Autodesk Inventor part; units mm, degrees
ref_plane "Work Plane1" through (-9, 0, 0) normal (1, 0, 0) x (0, 0, -1)
ref_plane "Work Plane2" through (-3.5, 4, 0) normal (0, 1, 0) x (1, 0, 0)
ref_plane "YZ Plane" through (0, 0, 0) normal (1, 0, 0) x (0, 1, 0)
sketch "Sketch1" plane through (0, 0, 0) normal (0, 1, 0) x (-1, 0, 0)
  line L0 (0, 0) -> (18, 0)
  line L1 (18, 0) -> (18, -4)
  line L2 (18, -4) -> (0, -4)
  line L3 (0, -4) -> (0, 0)
  line L4 (18, -2) -> (16, -2)
  line L5 (9, -4) -> (9, -3)
  circle A0 centre (16, -2) radius 1.1
  circle A1 centre (2, -2) radius 1.1
  dimension "d0" = 18
  dimension "d1" = 4
  dimension "d2" = 2
  dimension "d3" = 2.2
extrude "Extrusion1" add sketch "Sketch1" along normal blind 8 contours A0 | L0 L1 L2 L3 | A1
sketch "Sketch2" plane through (0, 0, -4) normal (0, 0, -1) x (-1, 0, 0)
  line L0 (18, 0) -> (18, 8)
  line L1 (18, 8) -> (18, 6.1)
  line L2 (18, 0) -> (0, 0)
  line L3 (18, 0) -> (18, 1.9)
  line L4 (18, 6.1) -> (14.5, 6.1)
  line L5 (14.5, 6.1) -> (14.5, 1.9)
  line L6 (14.5, 1.9) -> (18, 1.9)
  line L7 (18, 1.9) -> (18, 6.1)
  dimension "d6" = 1.9
  dimension "d7" = 1.9
  dimension "d8" = 3.5
extrude "Extrusion2" cut sketch "Sketch2" against normal blind 8
ref_plane "Work Plane1" through (-9, 0, 0) normal (1, 0, 0) x (0, 0, -1)
mirror "Mirror1" about plane through (-9, 0, 0) normal (1, 0, 0) of "Extrusion2"
extrude "Extrusion3" cut sketch "Sketch1" along normal blind 8 contours A0 | A1
sketch "Sketch4" plane through (0, 8, 0) normal (0, 1, 0) x (1, 0, 0)
  line L0 (-18, 0) -> (0, 0)
  line L1 (0, 0) -> (-4, 0)
  line L2 (-4, 0) -> (-4, 4)
  line L3 (-4, 4) -> (0, 4)
  line L4 (0, 4) -> (0, 0)
  circle A0 centre (-2, 2) radius 1.1
  circle A1 centre (-2, 2) radius 1.1
  dimension "d14" = 4
  dimension "d15" = 4
  dimension "d16" = 2.2
extrude "Extrusion4" add sketch "Sketch4" along normal blind 3.25
ref_plane "Work Plane2" through (-3.5, 4, 0) normal (0, 1, 0) x (1, 0, 0)
mirror "Mirror2" about plane through (-3.5, 4, 0) normal (0, 1, 0) of "Extrusion4"
fillet "Fillet2" radius 2 8 edges at (0, 8.675, -4) (0, -0.675, -4) (0, -0.675, 0) (0, 8.675, 0) (-18, 7.05, -4) (-18, 0.95, -4) (-18, 7.05, 0) (-18, 0.95, 0)
chamfer "Chamfer1" distance 3.25 angle 45 2 edges at (-4, 8, -2) (-4, 0, -2)
sketch "Sketch5" plane through (-14.5, 1.9, 0) normal (0, 0, 1) x (1, 0, 0)
  line L0 (0, 0) -> (-1.5, 0)
  line L1 (0, 0) -> (-4.1729, 0)
  line L2 (-4.1729, 0) -> (-4.1729, 7.3414)
  line L3 (-4.1729, 7.3414) -> (0, 7.3414)
  line L4 (0, 7.3414) -> (0, 0)
  line L5 (0, 0) -> (-4.2733, 0)
  line L6 (-4.2733, 0) -> (-4.2733, -4.4882)
  line L7 (-4.2733, -4.4882) -> (0, -4.4882)
  line L8 (0, -4.4882) -> (0, 0)
  point P0 (14.5, -1.9)
extrude "Extrusion5" cut sketch "Sketch5" against normal blind 10
sketch "Sketch6" plane through (0, 0, 0) normal (0, -1, 0) x (1, 0, 0)
  line L0 (-14.5, 0) -> (-14.5, -4)
  line L1 (-14.5, -2) -> (-16, -2)
  line L2 (-14.5, 0) -> (-7.25, 0)
  line L3 (-7.25, -4) -> (-14.5, -4)
  line L4 (-14.5, 0) -> (-12.5, 0)
  line L5 (-12.5, 0) -> (-12.5, -4)
  line L6 (-12.5, -4) -> (-14.5, -4)
  line L7 (-14.5, -4) -> (-14.5, 0)
  point P0 (0, 0)
  dimension "d25" = 1.5
  dimension "d26" = 2
extrude "Extrusion6" cut sketch "Sketch6" against normal blind 10
sketch "Sketch7" plane through (0, 0, 0) normal (0, -1, 0) x (1, 0, 0)
  line L0 (-12.5, 0) -> (-12.5, -4)
  line L1 (-12.5, -2) -> (-16, -2)
  line L2 (-12.5, 0) -> (-7.25, 0)
  line L3 (-16, -2) -> (-12.5, 0)
  line L4 (-7.25, -4) -> (-12.5, -4)
  line L5 (-12.5, 0) -> (-12.5, -4)
  line L6 (-12.5, -4) -> (-16, -2)
  point P0 (0, 0)
  dimension "d29" = 3.5
extrude "Extrusion7" add sketch "Sketch7" against normal blind 8
properties part number "short_link_v3"
Work out the finished part from the listing and answer in its coordinate system (mm). A direction names the side the tool comes from. Give positions to 0.01 mm unless a question says otherwise; leave off trailing zeros. Loops run counter-clockwise (first coordinate to the right, second up) from the corner with the lowest first, then second, coordinate; pieces in that order, holes last. Notation, with made-up numbers: (83.25, -35) - (94.25, -35) arc R22 ccw to (94.25, -13) - close; hole circle Ø7 at (49.25, 29). An arc over 180 degrees is marked (long way). Answer in a Markdown table with one row per item. Add a question column.
Q1. The part is cut by section C-C (x = -7.5). Determine the outline of the cut face in (y, z), and give its area (3 significant figures).
Q2. Each of these flat-tipped pins is pushed along its axis until it touches: P1, Ø2, axis at x = -11.5, z = -2, coming from the -Y side; P2, Ø1.5, axis at x = -7.5, y = 8.5, coming from the +Z side; P3, Ø1.8, axis at x = -2, z = -2, coming from the -Y side; P4, Ø1.5, axis at y = 5.5, z = -0.5, coming from the +X side. Where does it stop, or does it pass through?
Q3. The part is cut by section D-D (x = -13). Determine the outline of the cut face in (y, z), and give its area (3 significant figures).
Q4. A tool of negligible diameter and unlimited length cuts with its end or side. For faces 1 (the flat face through (-11, 8, -2)), 2 (the flat face through (-11, 0, -2)), 3 (the flat face through (-3, 11.25, -1)), 4 (the flat face through (-3.5, 4, -2)), 5 (the flat face through (-14.27, 3.94, -1.01)), from which of +Z, -Z, +X, -X, +Y, -Y can it reach the whole face along a straight path? Write none if from no direction.
Q5. Consider line 1 along Z through (x, y) = (-2, 0.75); line 2 along Y through (x, z) = (-9.75, -1); line 3 along X through (y, z) = (10.4, -2). Determine where each line is inside the solid, lowest interval first.
Q6. Determine the mould class of faces 6 (the cylindrical face through (-0.6, 8.71, -0.57)), 7 (the flat face through (-5.65, 9.6, -2.03)), 8 (the flat face through (-1, 6.1, -3)), 9 (the flat face through (-1, 1.9, -3)) for opening direction Y: released by +Y, released by -Y, zero draft, split by the parting line, or undercut.
Q7. The part is cut by section A-A (z = -2.5). State how many separate pieces and enclosed holes the cut face has, and give its area (3 significant figures).
Q8. The part is cut by section B-B (y = 3). Determine the outline of the cut face in (x, z).
Solution:
| question | item | result |
|---|---|---|
| 1 | outline | (0, -4) - (8, -4) - (8, 0) - (0, 0) - close |
| 1 | area | 32.0 mm² |
| 2 | P1 | stops at y = 0 |
| 2 | P2 | stops at z = 0 |
| 2 | P3 | passes through |
| 2 | P4 | stops at x = -0.3 |
| 3 | outline | (0, -3.71) - (8, -3.71) - (8, -0.29) - (0, -0.29) - close |
| 3 | area | 27.4 mm² |
| 4 | face 1 | +Z, -Z, -X, +Y |
| 4 | face 2 | +Z, -Z, -X, -Y |
| 4 | face 3 | +Z, -Z, +X, -X, +Y |
| 4 | face 4 | +Z, -Z, +X |
| 4 | face 5 | +Z, -X, +Y, -Y |
| 5 | line 1 | z = -4 to -3.1, -0.9 to 0 |
| 5 | line 2 | y = 0 to 8 |
| 5 | line 3 | x = -4.85 to -3.1, -0.9 to 0 |
| 6 | face 6 | zero draft |
| 6 | face 7 | released by +Y |
| 6 | face 8 | undercut |
| 6 | face 9 | undercut |
| 7 | separate pieces | 3 |
| 7 | enclosed holes | 0 |
| 7 | area | 122 mm² |
| 8 | outline | (-16, -2) - (-12.5, -4) - (-3.5, -4) - (-3.5, 0) - (-12.5, 0) - close |
